from build123d import *

# Parameters (mm, degrees)
SKETCH_1_R      = 2
SKETCH_1_W      = 40
SKETCH_1_H      = 40
SKETCH_1_R_2    = 1.5
SKETCH_1_R_3    = 19
EXTRUDE_1_DEPTH = 1


with BuildPart() as part:
    # Эскиз1 → Бобышка-Вытянуть1 (new body)
    # profile 1 of 2: a face of its own
    with BuildSketch(Plane(origin=(0, 0, 0), x_dir=(1, 0, 0), z_dir=(0, 1, 0))):
        with BuildLine():
            Line((-9, -28), (-9, -38))
            Line((-9, -38), (-23, -38))
            Line((-23, -38), (-23, 38))
            Line((-23, 38), (23, 38))
            Line((23, 38), (23, -38))
            Line((23, -38), (9, -38))
            Line((9, -38), (9, -28))
            ThreePointArc((9, -28), (0, -19), (-9, -28))
        make_face()
        with Locations(Location((15.4, -28, 0), (0, 0, 270))):
            Circle(SKETCH_1_R, mode=Mode.SUBTRACT)
        with Locations(Location((-15.4, -28, 0), (0, 0, 270))):
            Circle(SKETCH_1_R, mode=Mode.SUBTRACT)
        with Locations((0, 15)):
            Rectangle(SKETCH_1_W, SKETCH_1_H, mode=Mode.SUBTRACT)
    # profile 2 of 2: a face of its own
    with BuildSketch(Plane(origin=(0, 0, 0), x_dir=(1, 0, 0), z_dir=(0, 1, 0))):
        with Locations((0, 15)):
            Rectangle(SKETCH_1_W, SKETCH_1_H)
        with Locations(Location((-16.717514421, -1.717514421, 0), (0, 0, 270))):
            Circle(SKETCH_1_R_2, mode=Mode.SUBTRACT)
        with Locations(Location((16.717514421, -1.717514421, 0), (0, 0, 270))):
            Circle(SKETCH_1_R_2, mode=Mode.SUBTRACT)
        with Locations(Location((16.717514421, 31.717514421, 0), (0, 0, 270))):
            Circle(SKETCH_1_R_2, mode=Mode.SUBTRACT)
        with Locations(Location((-16.717514421, 31.717514421, 0), (0, 0, 270))):
            Circle(SKETCH_1_R_2, mode=Mode.SUBTRACT)
        with Locations(Location((0, 15, 0), (0, 0, 270))):
            Circle(SKETCH_1_R_3, mode=Mode.SUBTRACT)
    extrude(amount=EXTRUDE_1_DEPTH)


solid = part.part
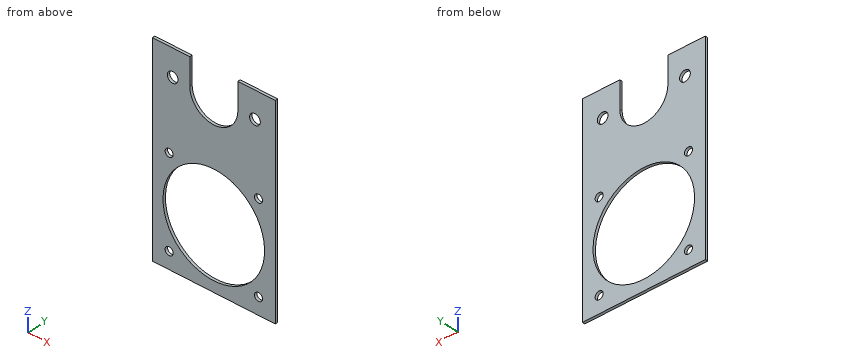
Design review of the part built by this model. Coordinates are the model's own, in mm. Round coordinates to 2 decimals unless told otherwise and drop trailing zeros. Write each loop counter-clockwise with the first axis right and the second up, starting at its lowest first coordinate (ties: lowest second). Pieces come first, ordered by that corner, then holes. Notation, with made-up numbers: (83.25, -24.5) - (121.25, -24.5) arc R9 ccw to (121.25, -17.5) - close; hole circle Ø6 at (51, 50.25). An arc over 180 degrees is marked (long way). Return JSON: item names as keys, results as strings. Group by question number.
Item 1: We need section C-C on y = 0.3. Write out the cut boundary in (x, z).
Item 2: We need section B-B on z = -15. Write out the cut boundary in (x, y).
Item 3: Insertion check: P1, Ø2.5, axis at x = -16.72, z = 1.72, coming from the -Y side. The pin has a flat end and moves straight along its axis. Give the tip position at first contact, or say it passes through.
Item 4: For probe 1 along X at (y, z) = (0.6, 28); probe 2 along X at (y, z) = (0.45, -15); probe 3 along Z at (x, y) = (15, 0.2), list the stretches that pass through material, from the lowest coordinate up. Write a range as [from, to].
Item 5: We need section A-A on x = 0. Write out the cut boundary in (y, z), and give its area (3 significant figures).
Model answer:
{
 "1": {"outline": "(-23, -38) - (23, -38) - (23, 38) - (9, 38) - (9, 28) arc R9 cw to (-9, 28) - (-9, 38) - (-23, 38) - close; hole circle Ø38 at (0, -15); hole circle Ø3 at (-16.72, -31.72); hole circle Ø3 at (-16.72, 1.72); hole circle Ø4 at (-15.4, 28); hole circle Ø4 at (15.4, 28); hole circle Ø3 at (16.72, -31.72); hole circle Ø3 at (16.72, 1.72)"},
 "2": {"outline": "(-23, 0) - (-19, 0) - (-19, 1) - (-23, 1) - close; (19, 0) - (23, 0) - (23, 1) - (19, 1) - close"},
 "3": {"P1": "passes through"},
 "4": {"probe 1": "x = [-23, -17.4], [-13.4, -9], [9, 13.4], [17.4, 23]", "probe 2": "x = [-23, -19], [19, 23]", "probe 3": "z = [-38, -26.66], [-3.34, 26.04], [29.96, 38]"},
 "5": {"outline": "(0, -38) - (1, -38) - (1, -34) - (0, -34) - close; (0, 4) - (1, 4) - (1, 19) - (0, 19) - close", "area": "19.0 mm²"}
}
